Source: CAD feature listing. Evaluate the final solid. Frame: model axes, mm. Face numbers are marked on the shaded views. Give positions to 0.01 mm unless a question says otherwise; leave off trailing zeros. Order: outer loops, then holes, each group sorted by start corner. A loop starts at its lowest first (then second) coordinate and runs counter-clockwise, first axis right, second up. Notation, with made-up numbers: (7.25, 36.25) - (37.25, 36.25) arc R27 ccw to (37.25, 70.25) - close; hole circle Ø7 at (76, 27). An arc over 180 degrees is marked (long way). Use CSV: the item, a comma, the result in double quotes.
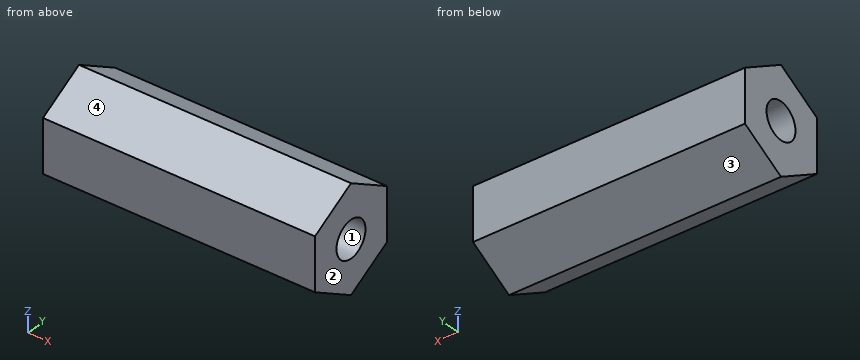
```python
from build123d import *

# Parameters (mm, degrees)
BOSS_EXTRUDE1_DEPTH     = 18.937499939
F_1_4_20_TAPPED_HOLE1_D = 5.1054


with BuildPart() as part:
    # Sketch1 → Boss-Extrude1 (new, symmetric)
    with BuildSketch(Plane(origin=(0, 0, 0), x_dir=(0, 0, -1), z_dir=(1, 0, 0))):
        Polygon((7.332348419, 0), (3.666174209, 6.35), (-3.666174209, 6.35), (-7.332348419, 0), (-3.666174209, -6.35), (3.666174209, -6.35), align=None)
    extrude(amount=BOSS_EXTRUDE1_DEPTH, both=True)

    # 1/4-20 Tapped Hole1 (through all)
    with Locations(Plane(origin=(18.937499939, 0, 0), x_dir=(0, 0, -1), z_dir=(1, 0, 0))):
        with Locations((0, 0)):
            Hole(F_1_4_20_TAPPED_HOLE1_D / 2)


solid = part.part
```
Item 1: Material intervals for line 1 (Y direction, x = 2.5, z = 0); line 2 (Y direction, x = -15.5, z = 0.75); line 3 (Z direction, x = -0.5, y = 0.75), sorted ascending. Write a range as from..to.
Filled in:
line 1,"y = -6.35..-2.55, 2.55..6.35"
line 2,"y = -6.35..-2.44, 2.44..6.35"
line 3,"z = -6.9..-2.44, 2.44..6.9"
Item 2: Section C-C on y = -3.75. Return the cut outline in (x, z).
Filled in:
outline,"(-18.94, -5.17) - (18.94, -5.17) - (18.94, 5.17) - (-18.94, 5.17) - close"
Item 3: Section A-A on z = 0. Return the cut outline in (x, y), then the cut area to 3 significant figures.
Filled in:
outline,"(-18.94, -6.35) - (18.94, -6.35) - (18.94, -2.55) - (-18.94, -2.55) - close; (-18.94, 2.55) - (18.94, 2.55) - (18.94, 6.35) - (-18.94, 6.35) - close"
area,"288 mm2"
Item 4: Section B-B on x = 14. Return the cut outline in (y, z).
Filled in:
outline,"(-6.35, -3.67) - (0, -7.33) - (6.35, -3.67) - (6.35, 3.67) - (0, 7.33) - (-6.35, 3.67) - close; hole circle Ø5.11 at (0, 0)"
Item 5: First-contact query: pin 1 (2 mm diameter, centred on x = -7.5, y = -2.5, fed in from +Z); pin 2 (1.5 mm diameter, centred on x = 0.5, y = 4.5, fed in from -Z); pin 3 (1.5 mm diameter, centred on x = -2.5, z = 5, fed in from +Y); pin 4 (4.5 mm diameter, centred on y = 0, z = 0, fed in from +X). Flat tips, straight axial feed; report the tip coordinate or a pass-through.
Filled in:
pin 1,"stops at z = 6.47"
pin 2,"stops at z = -5.17"
pin 3,"stops at y = 5.34"
pin 4,"passes through"
Item 6: Mould query, pull axis Z, two halves, no side actions, for the marked faces 1, 2, 3 and 4. Classes: released by +Z, released by -Z, zero draft, split by the parting line, or undercut.
Filled in:
face 1,"undercut"
face 2,"zero draft"
face 3,"released by -Z"
face 4,"released by +Z"
Item 7: Section D-D on z = -5.25. Return the cut outline in (x, y).
Filled in:
outline,"(-18.94, -3.61) - (18.94, -3.61) - (18.94, 3.61) - (-18.94, 3.61) - close"
